```python
from build123d import *

# Parameters (mm, degrees)
SKETCH2_W               = 98
SKETCH2_H               = 60
BOSS_EXTRUDE1_DEPTH     = 1
SKETCH3_W               = 98
SKETCH3_H               = 40
BOSS_EXTRUDE2_DEPTH     = 10
SKETCH4_R               = 2
CUT_EXTRUDE1_DEPTH      = 10
MIRROR2_COPY_1_SKETCH_R = 2
MIRROR2_COPY_1_DEPTH    = 10
SKETCH5_W               = 55
SKETCH5_H               = 20
BOSS_EXTRUDE3_DEPTH     = 10


with BuildPart() as part:
    # Sketch2 → Boss-Extrude1 (new body)
    with BuildSketch(Plane(origin=(0, 0, 0), x_dir=(1, 0, 0), z_dir=(0, 1, 0))):
        Rectangle(SKETCH2_W, SKETCH2_H)
    extrude(amount=BOSS_EXTRUDE1_DEPTH)

    # Sketch3 → Boss-Extrude2 (add)
    with BuildSketch(Plane(origin=(0, 1, 0), x_dir=(1, 0, 0), z_dir=(0, 1, 0))):
        Rectangle(SKETCH3_W, SKETCH3_H)
    extrude(amount=BOSS_EXTRUDE2_DEPTH)

    # Sketch4 → Cut-Extrude1 (cut)
    with BuildSketch(Plane(origin=(0, 1, 0), x_dir=(1, 0, 0), z_dir=(0, 1, 0))):
        with Locations(Location((-46, 27, 0), (0, 0, 270))):
            Circle(SKETCH4_R)
    cut_extrude1 = extrude(amount=-CUT_EXTRUDE1_DEPTH, mode=Mode.SUBTRACT)

    # Mirror1: Cut-Extrude1 across plane
    add(cut_extrude1.mirror(Plane.XY), mode=Mode.SUBTRACT)

    # Mirror2: Cut-Extrude1 across plane
    add(cut_extrude1.mirror(Plane(origin=(0, 0, 0), x_dir=(0, 0, 1), z_dir=(1, 0, 0))), mode=Mode.SUBTRACT)

    # Mirror2 copy 1 sketch → Mirror2 copy 1 (cut)
    with BuildSketch(Plane(origin=(0, 1, 0), x_dir=(-1, 0, 0), z_dir=(0, 1, 0))):
        with Locations(Location((-46, 27, 0), (0, 0, 270))):
            Circle(MIRROR2_COPY_1_SKETCH_R)
    extrude(amount=-MIRROR2_COPY_1_DEPTH, mode=Mode.SUBTRACT)

    # Sketch5 → Boss-Extrude3 (add)
    with BuildSketch(Plane.XZ):
        with Locations((21.5, 20)):
            Rectangle(SKETCH5_W, SKETCH5_H)
    extrude(amount=BOSS_EXTRUDE3_DEPTH)


solid = part.part
```
CAD build for the part. Positions are in the model's coordinates, mm. A direction names the side the tool comes from. Coordinates: 2 decimals unless noted, no trailing zeros. Write each loop counter-clockwise with the first axis right and the second up, starting at its lowest first coordinate (ties: lowest second). Pieces come first, ordered by that corner, then holes.
(1) 3-axis set-ups, long thin cutter, end or side, ignore diameter. For faces 5 (the face through (46, 0, 27)), 6 (the face through (-1, 6, -20)), 7 (the face through (47.774, 0.507, -26.077)), 8 (the face through (-1, 1, 25)): which of +Z, -Z, +X, -X, +Y, -Y reach the whole face in a straight line?
(2) Cut at D-D, the plane x = -46. List the corners of the cut face in (y, z).
(3) Cut at A-A, the plane z = -27. List the corners of the cut face in (x, y).
(4) Flat gauge pins, fed straight in: pin 1 (4.5 mm diameter, centred on x = 46, z = 26, fed in from +Y); pin 2 (2 mm diameter, centred on y = -1.5, z = 8.5, fed in from +X); pin 3 (5 mm diameter, centred on y = -3.5, z = 22, fed in from -X); pin 4 (5 mm diameter, centred on x = -7.5, y = 5.5, fed in from -Z). Where does each tip first touch, or does it go through?
(5) Cut at C-C, the plane z = 27. List the corners of the cut face in (x, y).
(6) Two-plate mould, pull along X, no slides. Class faces 1 (the face through (47.774, 0.507, 26.077)), 2 (the face through (-6, -5, 20)), 3 (the face through (49, 3, 6)), 4 (the face through (21, -5, 10)): +X half, -X half, draft (parallel to the pull), parting line (faces both ways), or undercut.
(7) Cut at B-B, the plane x = 46. List the corners of the cut face in (y, z).
(8) Drill centre lines: probe 1 along X at (y, z) = (0.6, 27); probe 2 along Z at (x, y) = (46, 0.65); probe 3 along Z at (x, y) = (-9, 3.5). Where is each one in solid material? Low to high.
Geometry says:
1. face 5: +Y
1. face 6: -Z, +X, -X, +Y
1. face 7: +Y, -Y
1. face 8: +Z, +X, -X, +Y
2. outline: (0, -30) - (1, -30) - (1, -29) - (0, -29) - close; (0, -25) - (1, -25) - (1, -20) - (11, -20) - (11, 20) - (1, 20) - (1, 25) - (0, 25) - close; (0, 29) - (1, 29) - (1, 30) - (0, 30) - close
3. outline: (-49, 0) - (-48, 0) - (-48, 1) - (-49, 1) - close; (-44, 0) - (44, 0) - (44, 1) - (-44, 1) - close; (48, 0) - (49, 0) - (49, 1) - (48, 1) - close
4. pin 1: stops at y = 1
4. pin 2: passes through
4. pin 3: stops at x = -6
4. pin 4: stops at z = -20
5. outline: (-49, 0) - (-48, 0) - (-48, 1) - (-49, 1) - close; (-44, 0) - (-6, 0) - (-6, -10) - (49, -10) - (49, 1) - (48, 1) - (48, 0) - (44, 0) - (44, 1) - (-44, 1) - close
6. face 1: undercut
6. face 2: -X half
6. face 3: +X half
6. face 4: draft
7. outline: (-10, 10) - (0, 10) - (0, -25) - (1, -25) - (1, -20) - (11, -20) - (11, 20) - (1, 20) - (1, 25) - (0, 25) - (0, 29) - (1, 29) - (1, 30) - (-10, 30) - close; (0, -30) - (1, -30) - (1, -29) - (0, -29) - close
8. probe 1: x = -49 to -48, -44 to 44, 48 to 49
8. probe 2: z = -30 to -29, -25 to 25, 29 to 30
8. probe 3: z = -20 to 20
